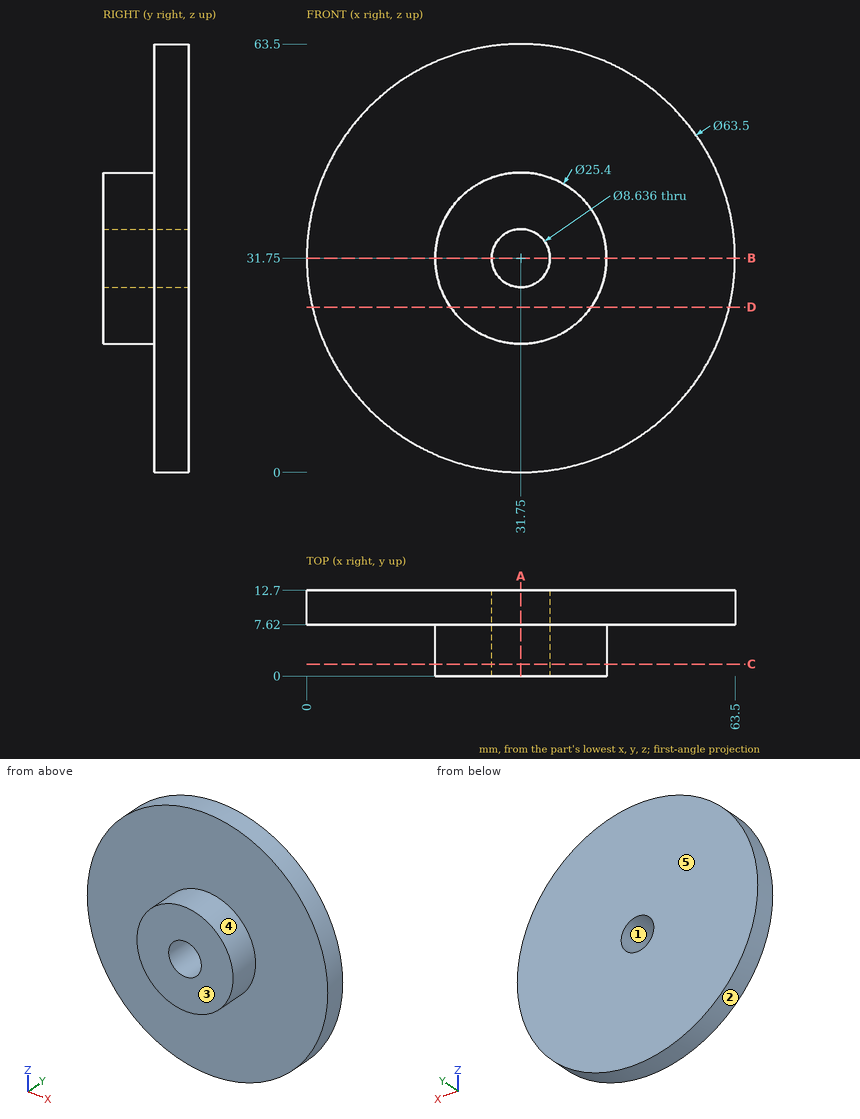
The figure shows three views and two pictorial views of one solid part (mm, origin at its lowest corner). Answer the questions. A direction names the side the tool comes from. Coordinates: 2 decimals unless noted, no trailing zeros. Loops run counter-clockwise (first coordinate to the right, second up) from the corner with the lowest first, then second, coordinate; pieces in that order, holes last. Notation, with made-up numbers: M -24.75,56 L 29.25,56 A26 ccw 29.25,93 Z; hole C -22,19.5 d2. An arc over 180 degrees is marked long. Answer as CSV lines item,"result". Start each with the question number.
(1) Find the intervals of material crossed by L1, parallel to Z at x = 31.75, y = 9.75; L2, parallel to X at y = 3, z = 32; L3, parallel to Y at x = 20.5, z = 44, in increasing order. Write a range as [from, to].
(2) The mould has two halves that part along Z. Classify the marked faces 1, 2 and 3: pulls with the +Z half, pulls with the -Z half, needs draft (parallel to the pull), parting line crosses it, or undercut.
(3) The part is cut by section D-D (z = 24.5). Give the vertices of the cut face in (x, y), and give its area (3 significant figures).
(4) The part is cut by section A-A (x = 31.75). Give the vertices of the cut face in (y, z).
(5) Given pin 1 (5 mm diameter, centred on x = 43.5, z = 40, fed in from -Y); pin 2 (7 mm diameter, centred on x = 31.75, z = 31.75, fed in from -Y), each flat-ended and moving along its own axis, determine where each tip first touches the part or whether it passes through.
(6) The part is cut by section B-B (z = 31.75). Give the vertices of the cut face in (x, y).
(7) For the marked faces 4 and 5, determine the directions among +Z, -Z, +X, -X, +Y, -Y from which every point of the face is accessible in a straight line to the end or side of a thin tool.
(8) The part is cut by section C-C (y = 1.75). Give the vertices of the cut face in (x, z), and give its area (3 significant figures).
Determined:
1,L1,"[0, 27.43], [36.07, 63.5]"
1,L2,"[19.05, 27.44], [36.06, 44.45]"
1,L3,"[7.62, 12.7]"
2,face 1,"undercut"
2,face 2,"parting line crosses it"
2,face 3,"needs draft"
3,outline,"M 0.84,7.62 L 21.32,7.62 L 21.32,0 L 42.18,0 L 42.18,7.62 L 62.66,7.62 L 62.66,12.7 L 0.84,12.7 Z"
3,area,"473 mm2"
4,outline,"M 0,19.05 L 7.62,19.05 L 7.62,0 L 12.7,0 L 12.7,27.43 L 0,27.43 Z; M 0,36.07 L 12.7,36.07 L 12.7,63.5 L 7.62,63.5 L 7.62,44.45 L 0,44.45 Z"
5,pin 1,"y = 0"
5,pin 2,"through"
6,outline,"M 0,7.62 L 19.05,7.62 L 19.05,0 L 27.43,0 L 27.43,12.7 L 0,12.7 Z; M 36.07,0 L 44.45,0 L 44.45,7.62 L 63.5,7.62 L 63.5,12.7 L 36.07,12.7 Z"
7,face 4,"-Y"
7,face 5,"+Z, -Z, +X, -X, +Y"
8,outline,"C 31.75,31.75 d25.4; hole C 31.75,31.75 d8.64"
8,area,"448 mm2"
